Work out the finished part from the listing and answer in its coordinate system (mm). A direction names the side the tool comes from. Give positions to 0.01 mm unless a question says otherwise; leave off trailing zeros. Order: outer loops, then holes, each group sorted by start corner. A loop starts at its lowest first (then second) coordinate and runs counter-clockwise, first axis right, second up.
```python
from build123d import *

# Parameters (mm, degrees)
EXTRUDE17_DEPTH = 1.6129
SKETCH19_R      = 3.6195
EXTRUDE19_DEPTH = 4.2291
SKETCH20_R      = 0.46355
SKETCH20_R_2    = 1.27
EXTRUDE20_DEPTH = 5.2291
SKETCH21_R      = 2.44475
EXTRUDE21_DEPTH = 1.1557
SKETCH22_R      = 2.286
EXTRUDE22_DEPTH = 2.3368


with BuildPart() as part:
    # Sketch18 → Extrude17 (new body)
    with BuildSketch(Plane(origin=(0, 0, 0), x_dir=(1, 0, 0), z_dir=(0, 1, 0))):
        with BuildLine():
            Line((-14.34305969, 1.923991942), (-2.13741415, 2.921))
            ThreePointArc((-2.13741415, 2.921), (3.6195, 0), (-2.13741415, -2.921))
            Line((-2.13741415, -2.921), (-14.34305969, -1.923991942))
            ThreePointArc((-14.34305969, -1.923991942), (-16.1163, 0), (-14.34305969, 1.923991942))
        make_face()
    extrude(amount=EXTRUDE17_DEPTH)

    # Sketch19 → Extrude19 (add)
    with BuildSketch(Plane(origin=(0, 1.6129, 0), x_dir=(1, 0, 0), z_dir=(0, 1, 0))):
        Circle(SKETCH19_R)
    extrude(amount=-EXTRUDE19_DEPTH)

    # Sketch20 → Extrude20 (cut, through all)
    with BuildSketch(Plane(origin=(0, 1.6129, 0), x_dir=(1, 0, 0), z_dir=(0, 1, 0))):
        with Locations((-14.1859, 0)):
            Circle(SKETCH20_R)
        Circle(SKETCH20_R_2)
        with Locations((-4.6609, 0)):
            Circle(SKETCH20_R)
        with Locations((-6.5659, 0)):
            Circle(SKETCH20_R)
        with Locations((-8.4709, 0)):
            Circle(SKETCH20_R)
        with Locations((-10.3759, 0)):
            Circle(SKETCH20_R)
        with Locations((-12.2809, 0)):
            Circle(SKETCH20_R)
    extrude(amount=-EXTRUDE20_DEPTH, mode=Mode.SUBTRACT)

    # Sketch21 → Extrude21 (cut)
    with BuildSketch(Plane(origin=(0, 1.6129, 0), x_dir=(1, 0, 0), z_dir=(0, 1, 0))):
        Circle(SKETCH21_R)
    extrude(amount=-EXTRUDE21_DEPTH, mode=Mode.SUBTRACT)

    # Sketch22 → Extrude22 (cut)
    with BuildSketch(Plane.XZ.offset(2.6162)):
        Circle(SKETCH22_R)
    extrude(amount=-EXTRUDE22_DEPTH, mode=Mode.SUBTRACT)


solid = part.part
```
1. The part is cut by section C-C (z = -1). Write down the section's boundary in (x, y).
Findings below:
outline: (-15.84, 0) - (-3.48, 0) - (-3.48, -2.62) - (-2.06, -2.62) - (-2.06, -0.28) - (-0.78, -0.28) - (-0.78, 0.46) - (-2.23, 0.46) - (-2.23, 1.61) - (-15.84, 1.61) - close; (0.78, -0.28) - (2.06, -0.28) - (2.06, -2.62) - (3.48, -2.62) - (3.48, 1.61) - (2.23, 1.61) - (2.23, 0.46) - (0.78, 0.46) - close
2. Given P1, Ø2, axis at y = -2, z = 2, coming from the -X side; P2, Ø1.5, axis at y = 0, z = -1, coming from the -X side, each flat-ended and moving along its own axis, determine where each tip first touches the part or whether it passes through.
Findings below:
P1: stops at x = -3.48
P2: stops at x = -16.1
3. Which of the six approach directions +Z, -Z, +X, -X, +Y, -Y give full straight-line access (tool end or side, diameter ignored) to faces 4 (the face through (-0.53, 1.043, 2.387)), 5 (the face through (-0.17, 0.09, -1.26)), 6 (the face through (-0.5, -1.46, -2.23))?
Findings below:
face 4: +Y
face 5: +Y, -Y
face 6: -Y
4. The part is cut by section A-A (x = 0). Write down the section's boundary in (y, z), then the cut area to 3 significant figures.
Findings below:
outline: (-2.62, -3.62) - (1.61, -3.62) - (1.61, -2.44) - (0.46, -2.44) - (0.46, -1.27) - (-0.28, -1.27) - (-0.28, -2.29) - (-2.62, -2.29) - close; (-2.62, 2.29) - (-0.28, 2.29) - (-0.28, 1.27) - (0.46, 1.27) - (0.46, 2.44) - (1.61, 2.44) - (1.61, 3.62) - (-2.62, 3.62) - close
area: 12.4 mm2
5. The part is cut by section B-B (y = 0.95). Write down the section's boundary in (x, z), then the cut area to 3 significant figures.
Findings below:
outline: (-14.34, -1.92) - (-2.14, -2.92) arc R3.62 ccw (long way) to (-2.14, 2.92) - (-14.34, 1.92) arc R1.93 ccw to start; hole circle Ø0.93 at (-14.19, 0); hole circle Ø0.93 at (-12.28, 0); hole circle Ø0.93 at (-10.38, 0); hole circle Ø0.93 at (-8.47, 0); hole circle Ø0.93 at (-6.57, 0); hole circle Ø0.93 at (-4.66, 0); hole circle Ø4.89 at (0, 0)
area: 76.7 mm2
6. Straight lines are drawn through the part: probe 1 along X at (y, z) = (-0.05, 0); probe 2 along Y at (x, z) = (-11, -2); probe 3 along Y at (x, z) = (-0.75, -1.75). For each, find the intervals that lie inside material, in ascending order.
Findings below:
probe 1: x = -3.62 to -1.27, 1.27 to 3.62
probe 2: y = 0 to 1.61
probe 3: y = -0.28 to 0.46
7. The part is cut by section D-D (z = 0). State how many separate pieces and enclosed holes the cut face has, then the cut area to 3 significant figures.
Findings below:
separate pieces: 8
enclosed holes: 0
area: 23.6 mm2
8. The mould has two halves that part along X. Classify faces 1 (the face through (-8.326, 0.795, -2.416)), 2 (the face through (-5.03, 0.82, 0.28)), 3 (the face through (-6, 1.613, 1)): pulls with the +X half, pulls with the -X half, needs draft (parallel to the pull), parting line crosses it, or undercut.
Findings below:
face 1: pulls with the -X half
face 2: undercut
face 3: needs draft
